Here's how the part is built. I have some questions about the finished solid (model axes, mm). Coordinates: 2 decimals unless noted, no trailing zeros. Write each loop counter-clockwise with the first axis right and the second up, starting at its lowest first coordinate (ties: lowest second). Pieces come first, ordered by that corner, then holes. Notation, with made-up numbers: (-8, -14) -> (4, -14) arc R27 ccw to (4, 4) -> close; hole circle Ø7 at (51, 85). An arc over 180 degrees is marked (long way). Put each result on its own line as item: value. Start each with the question number.
Item 1: I need wall thicknesses on line 1 (Y direction, x = -92.5, z = 4); line 2 (X direction, y = 2, z = 2.15); line 3 (X direction, y = 26.5, z = 3.7). Which ranges of each line are inside material? Lowest first, please. Write a range as [from, to].
Item 2: I want a section at A-A, the plane x = 0. List the corners of the cut face in (y, z) for me, then the cut area to 3 significant figures.
Item 3: If we mould it in two halves opening along Y, with no side actions, what happens to faces 1 (the face through (-2, -35, 3)), 2 (the face through (-2, 0, 0)), 3 (the face through (-0.7, 31.2, 3))? For each: released by +Y, released by -Y, zero draft, split by the parting line, or undercut.
from build123d import *

# Parameters (mm, degrees)
SKETCH_W        = 280
SKETCH_H        = 70
PAD_DEPTH       = 6
SKETCH001_R     = 5.1
SKETCH001_R_2   = 1.75
POCKET_DEPTH    = 6.001
SKETCH002_R     = 1.6
POCKET001_DEPTH = 583.360507
SKETCH003_W     = 24
SKETCH003_H     = 70
POCKET002_DEPTH = 6.001
FILLET_R        = 3


with BuildPart() as part:
    # Sketch → Pad (new body)
    with BuildSketch(Plane.XY):
        Rectangle(SKETCH_W, SKETCH_H)
    extrude(amount=PAD_DEPTH)

    # Sketch001 (on Face6 of Pad) → Pocket (cut, through all)
    with BuildSketch(Plane.XY.offset(6)):
        with Locations((0, 26.15)):
            Circle(SKETCH001_R)
        with Locations((-5.656854, 31.806854)):
            Circle(SKETCH001_R_2)
        with Locations((-5.656854, 20.493146)):
            Circle(SKETCH001_R_2)
        with Locations((5.656854, 31.806854)):
            Circle(SKETCH001_R_2)
        with Locations((5.656854, 20.493146)):
            Circle(SKETCH001_R_2)
    extrude(amount=-POCKET_DEPTH, mode=Mode.SUBTRACT)

    # Sketch002 (on Face5 of Pocket) → Pocket001 (cut, through all)
    with BuildSketch(Plane.XY.offset(6)):
        with Locations((-102.5, 2.5)):
            Circle(SKETCH002_R)
        with Locations((-92.5, 2.5)):
            Circle(SKETCH002_R)
    pocket001 = extrude(amount=-POCKET001_DEPTH, mode=Mode.SUBTRACT)

    # Mirrored: Pocket001 across Sketch002 V_Axis
    add(pocket001.mirror(Plane(origin=(0, 0, 6), x_dir=(0, 0, 1), z_dir=(1, 0, 0))), mode=Mode.SUBTRACT)

    # Sketch003 (on Face5 of Mirrored) → Pocket002 (cut, through all)
    with BuildSketch(Plane.XY.offset(6)):
        with Locations((-128, 0)):
            Rectangle(SKETCH003_W, SKETCH003_H)
        with Locations((128, 0)):
            Rectangle(SKETCH003_W, SKETCH003_H)
    extrude(amount=-POCKET002_DEPTH, mode=Mode.SUBTRACT)

    # Fillet
    fillet_edges = [part.edges().sort_by_distance(p)[0] for p in [
        (116, 35, 3),
        (116, -35, 3),
        (-116, 35, 3),
        (-116, -35, 3),
    ]]
    fillet(fillet_edges, radius=FILLET_R)


solid = part.part
Calculated:
1. line 1: y = [-35, 0.9], [4.1, 35]
1. line 2: x = [-116, -104.02], [-100.98, -94.02], [-90.98, 90.98], [94.02, 100.98], [104.02, 116]
1. line 3: x = [-116, -5.09], [5.09, 116]
2. outline: (-35, 0) -> (21.05, 0) -> (21.05, 6) -> (-35, 6) -> close; (31.25, 0) -> (35, 0) -> (35, 6) -> (31.25, 6) -> close
2. area: 359 mm2
3. face 1: released by -Y
3. face 2: zero draft
3. face 3: undercut
